Autodesk Inventor part; units mm, degrees
ref_plane "YZ Plane" through (0, 0, 0) normal (1, 0, 0) x (0, 1, 0)
ref_plane "XZ Plane" through (0, 0, 0) normal (0, 1, 0) x (-1, 0, 0)
ref_plane "XY Plane" through (0, 0, 0) normal (0, 0, 1) x (1, 0, 0)
sketch "Sketch1" plane through (0, 0, 0) normal (0, 0, 1) x (1, 0, 0)
  circle A0 centre (0, 0) radius 2.5
  line L0 (2.9774, 3.8259) -> (-2.9774, 3.8259)
  line L1 (-3.8259, 2.9774) -> (-3.8259, -2.9774)
  line L2 (-3.8259, -2.9774) -> (-8.8, -7.9515)
  line L3 (-7.9515, -8.8) -> (-2.9774, -3.8259)
  line L4 (2.9774, -3.8259) -> (7.9515, -8.8)
  line L5 (3.8259, 2.9774) -> (8.8, 7.9515)
  line L6 (8.8, -7.9515) -> (3.8259, -2.9774)
  line L7 (7.9515, 8.8) -> (2.9774, 3.8259)
  line L8 (-2.9774, 3.8259) -> (-7.9515, 8.8)
  line L9 (-8.8, 7.9515) -> (-3.8259, 2.9774)
  line L10 (-2.9774, -3.8259) -> (2.9774, -3.8259)
  line L11 (3.8259, -2.9774) -> (3.8259, 2.9774)
  line L12 (-3.1451, -8.8) -> (-2.6278, -10)
  line L13 (-3.1451, -8.8) -> (-7.9515, -8.8)
  line L14 (-10, -10) -> (-2.6278, -10)
  line L15 (2.6278, -10) -> (10, -10)
  line L16 (7.9515, -8.8) -> (3.1451, -8.7999)
  circle A1 centre (0, 0) radius 3.8259 construction
  line L17 (0, 0) -> (7.0677, 7.0677) construction
  circle A2 centre (2.7053, 2.7053) radius 1.1531 construction
  line L18 (-13.2321, 0) -> (16.76, 0) construction
  circle A3 centre (0, 0) radius 4.848 construction
  line L19 (2.6278, -10) -> (3.1451, -8.7999)
  line L20 (-8.8, -7.9515) -> (-8.8, -3.1451)
  line L21 (-8.8, -3.1451) -> (-10, -2.6278)
  line L22 (-8.8, 7.9515) -> (-8.8, 3.1451)
  line L23 (-8.8, 3.1451) -> (-10, 2.6278)
  line L24 (-7.9515, 8.8) -> (-3.1451, 8.8)
  line L25 (-3.1451, 8.8) -> (-2.6278, 10)
  line L26 (7.9515, 8.8) -> (3.1451, 8.8)
  line L27 (3.1451, 8.8) -> (2.6278, 10)
  line L28 (8.8, 7.9515) -> (8.8, 3.1451)
  line L29 (8.8, 3.1451) -> (10, 2.6278)
  line L30 (8.8, -7.9515) -> (8.8, -3.1451)
  line L31 (8.8, -3.1451) -> (10, -2.6278)
  line L32 (-10, 10) -> (-10, 2.6278)
  line L33 (-10, -2.6278) -> (-10, -10)
  line L34 (10, 10) -> (2.6278, 10)
  line L35 (-2.6278, 10) -> (-10, 10)
  line L36 (10, -10) -> (10, -2.6278)
  line L37 (10, 2.6278) -> (10, 10)
  point P0 (3.8259, 0)
  point P1 (-0.0241, 0)
  point P2 (-3.8259, 0)
  dimension "d3" = 20
  dimension "d4" = 20
  dimension "d5" = 5
  dimension "d10" = 1.2
  dimension "d12" = 1.2
  dimension "d13" = 1.2
  dimension "d14" = 1.2
  dimension "d16" = 20
  dimension "d17" = 1.2
  dimension "d18" = 1.2
  dimension "d19" = 1.2
  dimension "d20" = 1.2
  dimension "d21" = 1.2
  dimension "d22" = 20
extrude "Extrusion1" add sketch "Sketch1" along normal blind 240
fillet "Fillet1" radius 0.5 12 edges at (-8.8, 7.9515, 120) (-7.9515, 8.8, 120) (8.8, 7.9515, 120) (7.9515, 8.8, 120) (8.8, -7.9515, 120) (7.9515, -8.8, 120) (-7.9515, -8.8, 120) (-8.8, -7.9515, 120) (-10, -10, 120) (10, 10, 120) (-10, 10, 120) (10, -10, 120)
properties part number "240 beam"
Input: part model. Units: mm. Frame: model coordinates. A direction names the side the tool comes from. Give positions to 0.01 mm unless a question says otherwise; leave off trailing zeros. Write each loop counter-clockwise with the first axis right and the second up, starting at its lowest first coordinate (ties: lowest second). Pieces come first, ordered by that corner, then holes. Notation, with made-up numbers: M -20.75,34 L 1.25,34 A20 cw 1.25,72 Z; hole C 1,39 d10. An arc over 180 degrees is marked long. Write item = value, one per line. Start each with the question number.
1) Material intervals for line 1 along Y through (x, z) = (-6.25, 127.5); line 2 along X through (y, z) = (5, 41); line 3 along X through (y, z) = (6.5, 165), sorted ascending. Write a range as [from, to].
2) First-contact query: pin 1 Ø3 at (x, z) = (-1, 161) entering from +Y. Flat tip, straight axial feed; report the tip coordinate or a pass-through.
3) Draft query along X for faces 1 (the flat face through (-10, 6, 118)), 2 (the flat face through (6, 10, 118)), 3 (the flat face through (-5.01, 5.86, 118.32)). Return one class per face: +X half, -X half, draft (parallel to the pull), parting line (faces both ways), or undercut.
4) Reachability of faces 4 (the flat face through (-5.92, 5.07, 118.32)), 5 (the flat face through (-6, -10, 118)) from +Z, -Z, +X, -X, +Y, -Y: full face, straight path, thin tool, end or side. Return the list, or none.
5) Cut plane A-A on y = 0. Return the cut outline in (x, z), then the cut area to 3 significant figures.
Solved:
q1.line_1 = [-10, -8.8], [-7.1, -5.4], [5.4, 7.1], [8.8, 10]
q1.line_2 = [-10, -8.8], [-5.85, -4.15], [4.15, 5.85], [8.8, 10]
q1.line_3 = [-10, -8.8], [-7.35, -5.65], [5.65, 7.35], [8.8, 10]
q2.pin_1 = 3.83
q3.face_1 = -X half
q3.face_2 = draft
q3.face_3 = undercut
q4.face_4 = +Z, -Z
q4.face_5 = +Z, -Z, +X, -X, -Y
q5.outline = M -3.83,0 L -2.5,0 L -2.5,240 L -3.83,240 Z; M 2.5,0 L 3.83,0 L 3.83,240 L 2.5,240 Z
q5.area = 636 mm2
